Here's how the part is built. I have some questions about the finished solid (model axes, mm). Face numbers are marked on the shaded views. A direction names the side the tool comes from. Coordinates: 2 decimals unless noted, no trailing zeros. Write each loop counter-clockwise with the first axis right and the second up, starting at its lowest first coordinate (ties: lowest second). Pieces come first, ordered by that corner, then holes. Notation, with made-up numbers: (11.5, -22) -> (33.5, -22) arc R32 ccw to (33.5, 6) -> close; hole circle Ø2 at (27, 70). An arc over 180 degrees is marked (long way). Use a Markdown table: item, result. Add a question column.
Item 1: Will these pins go through, and if not, where does the flat tip stop? pin 1 Ø8 at (y, z) = (31.5, -5) entering from +X; pin 2 Ø2 at (x, z) = (13, 21) entering from -Y; pin 3 Ø1.5 at (y, z) = (-55, 3.5) entering from -X.
Item 2: If I drill on line 1 along Z through (x, y) = (-27.25, 0) (3 decimals); line 2 along Z through (x, y) = (8, 1); line 3 along Y through (x, z) = (-28.5, 8), over which ranges is the centre line in solid material (lowest first)? Write a range as from..to.
Item 3: Imagine slicing it at C-C, the plane z = 14. Write out the boundary of the cut face in (x, y).
Item 4: Imagine slicing it at D-D, the plane x = 7. Write out the boundary of the cut face in (y, z) (3 decimals), and give its area (3 significant figures).
Item 5: Imagine slicing it at B-B, the plane x = -25.5. Write out the boundary of the cut face in (y, z) (3 decimals), and give its area (3 significant figures).
Item 6: If we mould it in two halves opening along Y, with no side actions, what happens to the marked faces 4 and 5? For each: pulls with the +Y half, pulls with the -Y half, needs draft (parallel to the pull), parting line crosses it, or undercut.
Item 7: On a 3-axis mill with a long thin cutter (end or side, diameter ignored), from which of +Z, -Z, +X, -X, +Y, -Y can I reach the whole of each face in a straight line? I mean the marked faces 1, 2 and 3. Say none if no direction works.
Item 8: Imagine slicing it at A-A, the plane y = 0. Write out the boundary of the cut face in (x, z) (3 decimals), and give its area (3 significant figures).
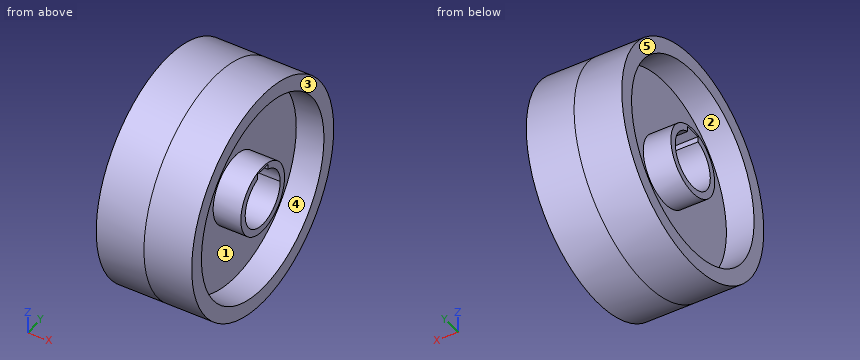
Solid Edge part; units mm, degrees
sketch "Sketch1" plane through (0, 0, 0) normal (1, 0, 0) x (0, 1, 0)
  circle A0 centre (0, 0) radius 20
  circle A1 centre (0, 0) radius 81.125
extrude "Protrusion1" add sketch "Sketch1" along normal mid plane 69
sketch "Sketch2" plane through (34.5, 0, 0) normal (1, 0, 0) x (0, 1, 0)
  circle A0 centre (0, 0) radius 70
  circle A1 centre (0, 0) radius 25
extrude "VaciadoExtruido_1" cut sketch "Sketch2" against normal blind 20
mirror "Mirror1" about plane through (0, 0, 0) normal (1, 0, 0) of "VaciadoExtruido_1"
sketch "Sketch3" plane through (34.5, 0, 0) normal (1, 0, 0) x (0, 1, 0)
  line L0 (-6, 23.1) -> (-6, 19.0788)
  line L1 (6, 23.1) -> (6, 19.0788)
  line L2 (0, 23.1) -> (6, 23.1)
  line L3 (0, 23.1) -> (-6, 23.1)
  arc A0 (-6, 19.0788) -> (6, 19.0788) centre (0, 0) cw
extrude "Cutout2" cut sketch "Sketch3" along normal mid plane 200
properties material "Acero"
Ans:
| question | item | result |
|---|---|---|
| 1 | pin 1 | stops at x = 14.5 |
| 1 | pin 2 | stops at y = -78.62 |
| 1 | pin 3 | stops at x = -14.5 |
| 2 | line 1 | z = -81.125..-70, -25..-20, 23.1..25, 70..81.125 |
| 2 | line 2 | z = -81.12..-19.97, 23.1..81.12 |
| 2 | line 3 | y = -80.73..-69.54, -23.69..-18.33, 18.33..23.69, 69.54..80.73 |
| 3 | outline | (-34.5, -79.91) -> (34.5, -79.91) -> (34.5, -68.59) -> (14.5, -68.59) -> (14.5, -20.71) -> (34.5, -20.71) -> (34.5, -14.28) -> (-34.5, -14.28) -> (-34.5, -20.71) -> (-14.5, -20.71) -> (-14.5, -68.59) -> (-34.5, -68.59) -> close; (-34.5, 14.28) -> (34.5, 14.28) -> (34.5, 20.71) -> (14.5, 20.71) -> (14.5, 68.59) -> (34.5, 68.59) -> (34.5, 79.91) -> (-34.5, 79.91) -> (-34.5, 68.59) -> (-14.5, 68.59) -> (-14.5, 20.71) -> (-34.5, 20.71) -> close |
| 4 | outline | circle Ø162.25 at (0, 0); hole (-6, 19.079) arc R20 ccw (long way) to (6, 19.079) -> (6, 23.1) -> (-6, 23.1) -> close |
| 4 | area | 19,400 mm^2 |
| 5 | outline | circle Ø162.25 at (0, 0); circle Ø50 at (0, 0); hole circle Ø140 at (0, 0); hole (-6, 19.079) arc R20 ccw (long way) to (6, 19.079) -> (6, 23.1) -> (-6, 23.1) -> close |
| 5 | area | 5,950 mm^2 |
| 6 | face 4 | undercut |
| 6 | face 5 | needs draft |
| 7 | face 1 | +X |
| 7 | face 2 | -X |
| 7 | face 3 | +Z, -Z, +X, +Y, -Y |
| 8 | outline | (-34.5, -81.125) -> (34.5, -81.125) -> (34.5, -70) -> (14.5, -70) -> (14.5, -25) -> (34.5, -25) -> (34.5, -20) -> (-34.5, -20) -> (-34.5, -25) -> (-14.5, -25) -> (-14.5, -70) -> (-34.5, -70) -> close; (-34.5, 23.1) -> (34.5, 23.1) -> (34.5, 25) -> (14.5, 25) -> (14.5, 70) -> (34.5, 70) -> (34.5, 81.125) -> (-34.5, 81.125) -> (-34.5, 70) -> (-14.5, 70) -> (-14.5, 25) -> (-34.5, 25) -> close |
| 8 | area | 4,620 mm^2 |
